CAD build for the part. Positions are in the model's coordinates, mm. Face numbers are marked on the shaded views. A direction names the side the tool comes from. Give positions to 0.01 mm unless a question says otherwise; leave off trailing zeros. Write each loop counter-clockwise with the first axis right and the second up, starting at its lowest first coordinate (ties: lowest second). Pieces come first, ordered by that corner, then holes. Notation, with made-up numbers: (-7.5, 28) -> (43.5, 28) arc R22 cw to (43.5, 60) -> close; hole circle Ø4 at (42, -7). An arc over 180 degrees is marked (long way). Answer in a Markdown table with one row per item. Add a question column.
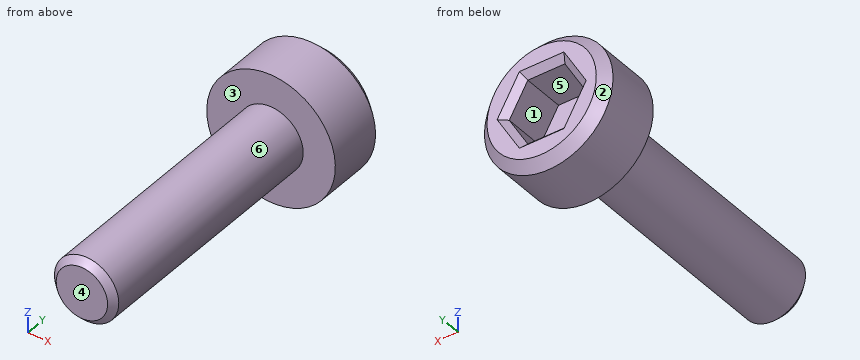
```python
from build123d import *

# Parameters (mm, degrees)
SKETCH1_R           = 2
BOSS_EXTRUDE1_DEPTH = 2
CHAMFER1_SIZE       = 0.3
CUT_EXTRUDE1_DEPTH  = 1.5
CHAMFER2_SIZE       = 0.2
SKETCH3_R           = 1
BOSS_EXTRUDE2_DEPTH = 8
CHAMFER3_SIZE       = 0.2


with BuildPart() as part:
    # Sketch1 → Boss-Extrude1 (new body)
    with BuildSketch(Plane(origin=(0, 0, 0), x_dir=(1, 0, 0), z_dir=(0, 1, 0))):
        with Locations(Location((0, 0, 0), (0, 0, 270))):  # turned: the seam where the file's is
            Circle(SKETCH1_R)
    extrude(amount=BOSS_EXTRUDE1_DEPTH)

    # Chamfer1
    chamfer1_edges = [part.edges().sort_by_distance(p)[0] for p in [
        (0, 2, -2),
    ]]
    chamfer(chamfer1_edges, length=CHAMFER1_SIZE)

    # Sketch2 → Cut-Extrude1 (cut)
    with BuildSketch(Plane(origin=(0, 2, 0), x_dir=(1, 0, 0), z_dir=(0, 1, 0))):
        Polygon((1.154700538, 0), (0.577350269, 1), (-0.577350269, 1), (-1.154700538, 0), (-0.577350269, -1), (0.577350269, -1), align=None)
    extrude(amount=-CUT_EXTRUDE1_DEPTH, mode=Mode.SUBTRACT)

    # Chamfer2
    chamfer2_edges = [part.edges().sort_by_distance(p)[0] for p in [
        (0.866025404, 2, 0.5),
        (0.866025404, 2, -0.5),
        (0, 2, -1),
        (-0.866025404, 2, -0.5),
        (-0.866025404, 2, 0.5),
        (0, 2, 1),
    ]]
    chamfer(chamfer2_edges, length=CHAMFER2_SIZE)

    # Sketch3 → Boss-Extrude2 (add)
    with BuildSketch(Plane.XZ):
        with Locations(Location((0, 0, 0), (0, 0, 90))):  # turned: the seam where the file's is
            Circle(SKETCH3_R)
    extrude(amount=BOSS_EXTRUDE2_DEPTH)

    # Chamfer3
    chamfer3_edges = [part.edges().sort_by_distance(p)[0] for p in [
        (0, -8, -1),
    ]]
    chamfer(chamfer3_edges, length=CHAMFER3_SIZE)


solid = part.part
```
Item 1: Slice it at A-A, the plane x = 0. List the corners of the cut face in (y, z), then the cut area to 3 significant figures.
Item 2: Which spindle directions (+Z, -Z, +X, -X, +Y, -Y) get a long thin tool onto all of the face, cutting with end or side? Do the marked faces 4, 5 and 6. Say none if no direction does.
Item 3: Probe L1, parallel to Y at x = -0.75, z = 0.2; L2, parallel to Z at x = 0.7, y = 1.75; L3, parallel to X at y = 1, z = -0.55. List the from-to ranges inside material, lowest first. Write a range as from..to.
Item 4: Drop a flat-ended pin along its axis: pin 1 Ø1 at (y, z) = (-2, 0.5) entering from -X. Give the stop position or say it passes through.
Item 5: Mould opens along Z. For the marked faces 1, 2 and 3 say: released by +Z, released by -Z, zero draft, split by the parting line, or undercut.
Item 6: Slice it at B-B, the plane y = 0.75. List the corners of the cut face in (x, z), then the cut area to 3 significant figures.
Item 7: Slice it at C-C, the plane y = -4. List the corners of the cut face in (x, z).
Answer key:
| question | item | result |
|---|---|---|
| 1 | outline | (-8, -0.8) -> (-7.8, -1) -> (0, -1) -> (0, -2) -> (1.7, -2) -> (2, -1.7) -> (2, -1.2) -> (1.8, -1) -> (0.5, -1) -> (0.5, 1) -> (1.8, 1) -> (2, 1.2) -> (2, 1.7) -> (1.7, 2) -> (0, 2) -> (0, 1) -> (-7.8, 1) -> (-8, 0.8) -> close |
| 1 | area | 20.8 mm² |
| 2 | face 4 | +Z, -Z, +X, -X, -Y |
| 2 | face 5 | +Y |
| 2 | face 6 | -Y |
| 3 | L1 | y = -8..0.5 |
| 3 | L2 | z = -1.82..-0.79, 0.79..1.82 |
| 3 | L3 | x = -1.92..-0.84, 0.84..1.92 |
| 4 | pin 1 | stops at x = -1 |
| 5 | face 1 | undercut |
| 5 | face 2 | split by the parting line |
| 5 | face 3 | zero draft |
| 6 | outline | circle Ø4 at (0, 0); hole (-1.15, 0) -> (-0.58, -1) -> (0.58, -1) -> (1.15, 0) -> (0.58, 1) -> (-0.58, 1) -> close |
| 6 | area | 9.10 mm² |
| 7 | outline | circle Ø2 at (0, 0) |
